Can you work these out from the drawing? Everything is in mm from the part's minimum corner. A direction names the side the tool comes from. Coordinates: 2 decimals unless noted, no trailing zeros. Order: outer loops, then holes, each group sorted by start corner. A loop starts at its lowest first (then second) coordinate and runs counter-clockwise, first axis right, second up. Notation, with made-up numbers: (-29.75, -38.5) -> (6.25, -38.5) arc R26 cw to (6.25, -19.5) -> close; hole circle Ø1 at (28, -34.5). An arc over 180 degrees is marked (long way). Write item = value, one per line. Start each with the question number.
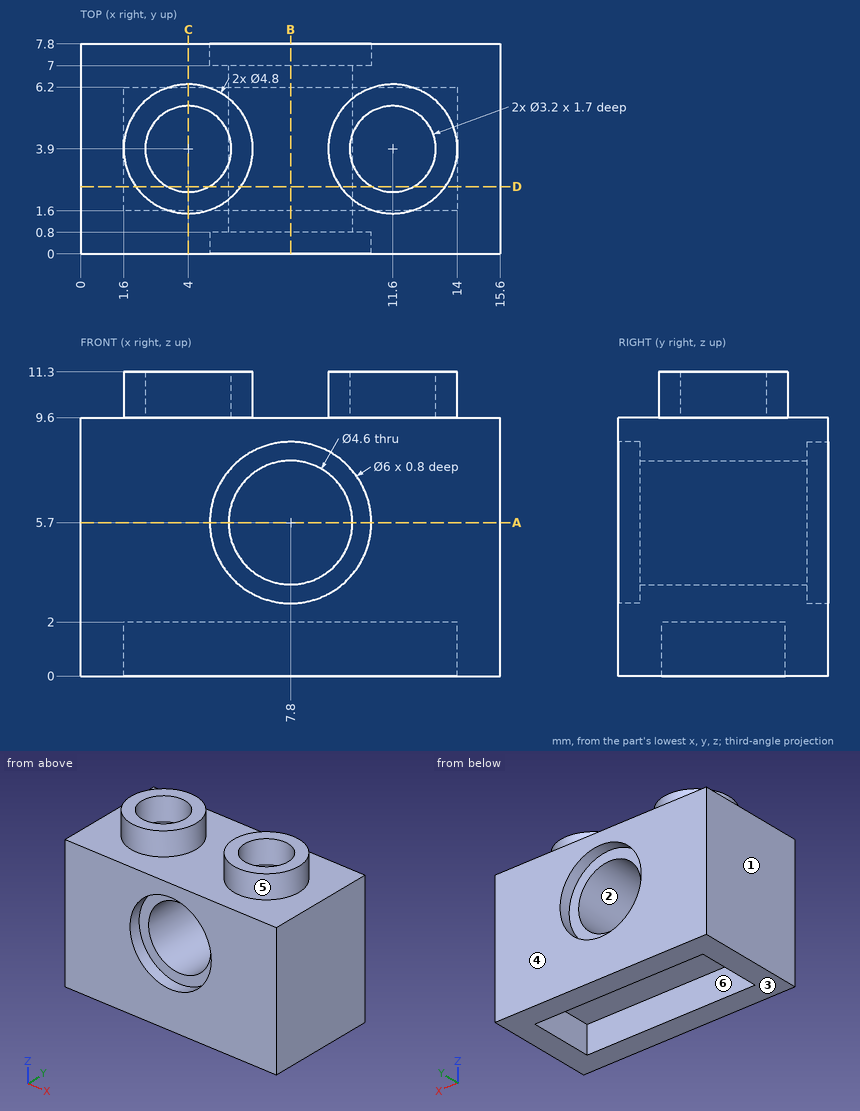
(1) If I drill on L1, parallel to Z at x = 7.8, y = 7.5; L2, parallel to X at y = 5.5, z = 1.5; L3, parallel to Y at x = 11.5, z = 10.25, over which ranges is the centre line in solid material (lowest first)? Write a range as from..to.
(2) For P1, Ø5.5, axis at x = 7.8, z = 5.7, coming from the +Y side; P2, Ø3, axis at y = 5.5, z = 7, coming from the -X side; P3, Ø2.5, axis at x = 6, y = 3.5, coming from the -Z side, each with a flat end and sliding along its axis, tell me the tip position at first contact or that it passes through.
(3) For the marked faces 4, 5 and 6, which set-ups out of +Z, -Z, +X, -X, +Y, -Y let a thin tool reach every point of the face, with its end or its side?
(4) Imagine slicing it at A-A (z = 5.7). Write out the boundary of the cut face in (x, y), plus the area to 3 significant figures.
(5) Thinking about a two-plate mould opening in Z: for the marked faces 1, 2 and 3, which applies, +Z half, -Z half, draft (parallel to the pull), parting line (faces both ways), or undercut?
(6) Imagine slicing it at C-C (x = 4). Write out the boundary of the cut face in (y, z), plus the area to 3 significant figures.
(7) Imagine slicing it at B-B (x = 7.8). Write out the boundary of the cut face in (y, z), plus the area to 3 significant figures.
(8) Imagine slicing it at D-D (y = 2.5). Write out the boundary of the cut face in (x, z).
Result set:
q1.L1 = 0..2.7, 8.7..9.6
q1.L2 = 0..1.6, 14..15.6
q1.L3 = 1.5..2.3, 5.5..6.3
q2.P1 = 7
q2.P2 = 0
q2.P3 = 2
q3.face_4 = +Z, -Z, +X, -X, +Y
q3.face_5 = +Z
q3.face_6 = -Z
q4.outline = (0, 0) -> (4.8, 0) -> (4.8, 0.8) -> (5.5, 0.8) -> (5.5, 7) -> (4.8, 7) -> (4.8, 7.8) -> (0, 7.8) -> close; (10.1, 0.8) -> (10.8, 0.8) -> (10.8, 0) -> (15.6, 0) -> (15.6, 7.8) -> (10.8, 7.8) -> (10.8, 7) -> (10.1, 7) -> close
q4.area = 83.6 mm2
q5.face_1 = draft
q5.face_2 = undercut
q5.face_3 = -Z half
q6.outline = (0, 0) -> (1.6, 0) -> (1.6, 2) -> (6.2, 2) -> (6.2, 0) -> (7.8, 0) -> (7.8, 9.6) -> (6.3, 9.6) -> (6.3, 11.3) -> (5.5, 11.3) -> (5.5, 9.6) -> (2.3, 9.6) -> (2.3, 11.3) -> (1.5, 11.3) -> (1.5, 9.6) -> (0, 9.6) -> close
q6.area = 68.4 mm2
q7.outline = (0, 0) -> (1.6, 0) -> (1.6, 2) -> (6.2, 2) -> (6.2, 0) -> (7.8, 0) -> (7.8, 2.7) -> (7, 2.7) -> (7, 3.4) -> (0.8, 3.4) -> (0.8, 2.7) -> (0, 2.7) -> close; (0, 8.7) -> (0.8, 8.7) -> (0.8, 8) -> (7, 8) -> (7, 8.7) -> (7.8, 8.7) -> (7.8, 9.6) -> (0, 9.6) -> close
q7.area = 27.6 mm2
q8.outline = (0, 0) -> (1.6, 0) -> (1.6, 2) -> (14, 2) -> (14, 0) -> (15.6, 0) -> (15.6, 9.6) -> (13.55, 9.6) -> (13.55, 11.3) -> (12.37, 11.3) -> (12.37, 9.6) -> (10.83, 9.6) -> (10.83, 11.3) -> (9.65, 11.3) -> (9.65, 9.6) -> (5.95, 9.6) -> (5.95, 11.3) -> (4.77, 11.3) -> (4.77, 9.6) -> (3.23, 9.6) -> (3.23, 11.3) -> (2.05, 11.3) -> (2.05, 9.6) -> (0, 9.6) -> close; hole circle Ø4.6 at (7.8, 5.7)
